```python
from build123d import *

# Parameters (mm, degrees)
F1_DEPTH = 25.4
F2_W     = 10.244804
F2_H     = 5.900593
F3_DEPTH = 12.7
F4_DEPTH = 12.7
F5_W     = 11.174377
F5_H     = 8.899484
F6_DEPTH = 25.4


with BuildPart() as f1:
    # F0 (on Front) → F1 (new body)
    with BuildSketch(Plane.XZ):
        Polygon((11.595629, 31.75), (11.595629, 0), (36.995629, 0), (36.995629, 31.75), (30.645629, 31.75), (30.645629, 22.77716), (17.945629, 22.77716), (17.945629, 31.75), align=None)
    extrude(amount=F1_DEPTH)

    # F2 (on Right) → F3 (cut)
    with BuildSketch(Plane.YZ):
        with Locations((-12.251601, 2.950296)):
            Rectangle(F2_W, F2_H)
    extrude(amount=-F3_DEPTH, mode=Mode.SUBTRACT)

    # F2 (on Right) → F4 (cut)
    with BuildSketch(Plane.YZ):
        with Locations((-12.251601, 2.950296)):
            Rectangle(F2_W, F2_H)
    extrude(amount=-F4_DEPTH, mode=Mode.SUBTRACT)

    # F5 (on face) → F6 (cut)
    with BuildSketch(Plane(origin=(11.595629, 0, 0), x_dir=(0, -1, 0), z_dir=(-1, 0, 0))):
        with Locations((10.92072, 4.449742)):
            Rectangle(F5_W, F5_H)
    extrude(amount=-F6_DEPTH, mode=Mode.SUBTRACT)


solid = f1.part
```
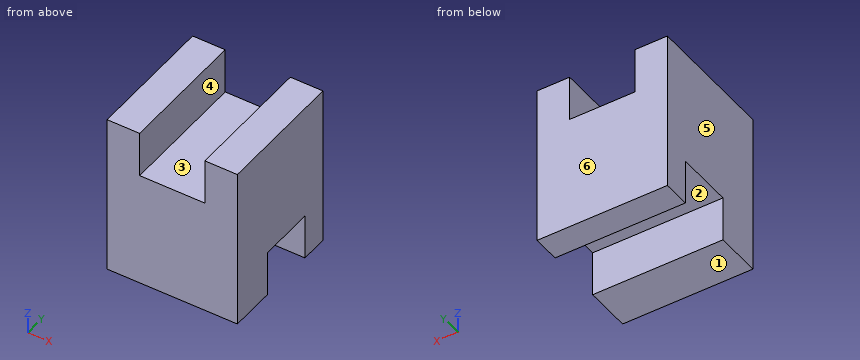
Input: part model. Units: mm. Frame: model coordinates. Face numbers are marked on the shaded views. A direction names the side the tool comes from. Give positions to 0.01 mm unless a question says otherwise; leave off trailing zeros. Order: outer loops, then holes, each group sorted by start corner. A loop starts at its lowest first (then second) coordinate and runs counter-clockwise, first axis right, second up.
1. Draft query along X for the marked faces 4, 5 and 6. Return one class per face: released by +X, released by -X, zero draft, split by the parting line, or undercut.
Computed:
face 4: undercut
face 5: released by -X
face 6: zero draft
2. Line query: probe 1 along X at (y, z) = (-17.5, 24); probe 2 along Y at (x, z) = (32.5, 4); probe 3 along Z at (x, y) = (25, -11.5). Output: solid intervals per line, ascending.
Computed:
probe 1: x = 11.6 to 17.95, 30.65 to 37
probe 2: y = -25.4 to -16.51, -5.33 to 0
probe 3: z = 8.9 to 22.78
3. Cut plane A-A (z = 3.5). Return loops of the section in (x, y), and give its area (3 significant figures).
Computed:
outline: (11.6, -25.4) - (37, -25.4) - (37, -16.51) - (11.6, -16.51) - close; (11.6, -5.33) - (37, -5.33) - (37, 0) - (11.6, 0) - close
area: 361 mm2
4. Cut plane D-D (z = 23.5). Return loops of the section in (x, y).
Computed:
outline: (11.6, -25.4) - (17.95, -25.4) - (17.95, 0) - (11.6, 0) - close; (30.65, -25.4) - (37, -25.4) - (37, 0) - (30.65, 0) - close
5. Cut plane B-B (x = 35). Return loops of the section in (y, z).
Computed:
outline: (-25.4, 0) - (-16.51, 0) - (-16.51, 8.9) - (-5.33, 8.9) - (-5.33, 0) - (0, 0) - (0, 31.75) - (-25.4, 31.75) - close
6. Set-up query: the marked faces 1, 2 and 3. Return all of +Z, -Z, +X, -X, +Y, -Y with unobstructed straight access to the full face (end or side cutting, diameter ignored); none if empty.
Computed:
face 1: -Z, +X, -X, +Y, -Y
face 2: -Z, +X, -X
face 3: +Z, +Y, -Y
7. Cut plane C-C (y = -18.5). Return loops of the section in (x, z), and give its area (3 significant figures).
Computed:
outline: (11.6, 0) - (37, 0) - (37, 31.75) - (30.65, 31.75) - (30.65, 22.78) - (17.95, 22.78) - (17.95, 31.75) - (11.6, 31.75) - close
area: 692 mm2
8. Pin query (flat end, axial travel): pin 1 Ø2 at (x, y) = (32, -13.5) entering from -Z; pin 2 Ø2.5 at (x, z) = (26.5, 4) entering from +Y; pin 3 Ø1.5 at (x, y) = (23.5, -7) entering from +Z. Return the tip coordinate at first contact, or that it passes through.
Computed:
pin 1: stops at z = 8.9
pin 2: stops at y = 0
pin 3: stops at z = 22.78
